```python
from build123d import *

# Parameters (mm, degrees)
SKETCH1_W                = 26.92
SKETCH1_H                = 12.7
BOSS_EXTRUDE1_DEPTH      = 4.95
BOSS_EXTRUDE1_DEPTH_BACK = 3.56
CUT_EXTRUDE1_DEPTH       = 9.51
SKETCH3_R                = 2.425
BOSS_EXTRUDE2_DEPTH      = 20.57
FILLET1_R                = 2.425
CHAMFER1_SIZE            = 0.5


with BuildPart() as part:
    # Sketch1 → Boss-Extrude1 (new body, two sides)
    with BuildSketch(Plane.XY) as boss_extrude1_sk:
        Rectangle(SKETCH1_W, SKETCH1_H)
    extrude(amount=BOSS_EXTRUDE1_DEPTH)
    extrude(boss_extrude1_sk.sketch, amount=-BOSS_EXTRUDE1_DEPTH_BACK)

    # Sketch2 → Cut-Extrude1 (cut, through all)
    with BuildSketch(Plane.XY.offset(4.95)):
        with BuildLine():
            Line((-12.065, 1.825), (-13.46, 1.825))
            ThreePointArc((-13.46, 1.825), (-14.425, 2.79), (-13.46, 3.755))
            Line((-13.46, 3.755), (-12.065, 3.755))
            ThreePointArc((-12.065, 3.755), (-11.1, 2.79), (-12.065, 1.825))
        make_face()
        with BuildLine():
            Line((12.065, 1.825), (13.46, 1.825))
            ThreePointArc((13.46, 1.825), (14.425, 2.79), (13.46, 3.755))
            Line((13.46, 3.755), (12.065, 3.755))
            ThreePointArc((12.065, 3.755), (11.1, 2.79), (12.065, 1.825))
        make_face()
    extrude(amount=-CUT_EXTRUDE1_DEPTH, mode=Mode.SUBTRACT)

    # Sketch3 → Boss-Extrude2 (add)
    with BuildSketch(Plane(origin=(13.46, 0, 0), x_dir=(0, 0, -1), z_dir=(1, 0, 0))):
        with Locations((0, -2.79)):
            Circle(SKETCH3_R)
    extrude(amount=BOSS_EXTRUDE2_DEPTH)

    # Fillet1
    fillet1_edges = [part.edges().sort_by_distance(p)[0] for p in [
        (34.03, -2.79, 2.425),
    ]]
    fillet(fillet1_edges, radius=FILLET1_R)

    # Chamfer1
    chamfer1_edges = [part.edges().sort_by_distance(p)[0] for p in [
        (13.46, 6.35, 0.695),
        (13.46, 5.0525, -3.56),
        (0, 6.35, -3.56),
        (-13.46, 6.35, 0.695),
        (13.46, 5.0525, 4.95),
        (0, 6.35, 4.95),
        (-13.46, 5.0525, 4.95),
        (13.46, -6.35, 0.695),
        (-13.46, -2.2625, -3.56),
        (13.46, -2.2625, -3.56),
        (0, -6.35, -3.56),
        (-13.46, -6.35, 0.695),
        (13.46, -2.2625, 4.95),
        (0, -6.35, 4.95),
        (-13.46, -2.2625, 4.95),
    ]]
    chamfer(chamfer1_edges, length=CHAMFER1_SIZE)


solid = part.part
```
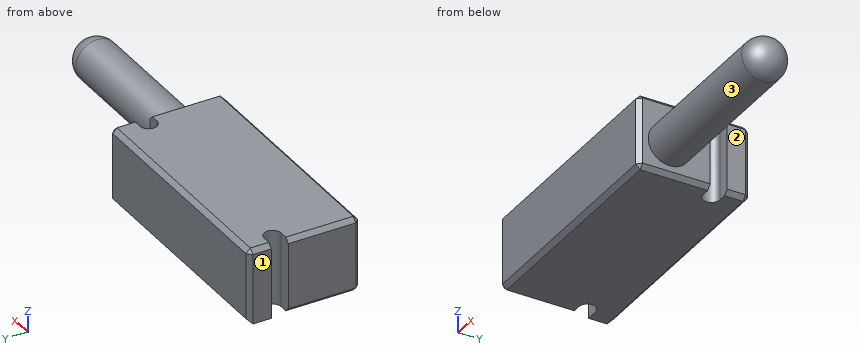
CAD build for the part. Positions are in the model's coordinates, mm. Face numbers are marked on the shaded views. A direction names the side the tool comes from. Round coordinates to 2 decimals unless told otherwise and drop trailing zeros. Order: outer loops, then holes, each group sorted by start corner. A loop starts at its lowest first (then second) coordinate and runs counter-clockwise, first axis right, second up. Notation, with made-up numbers: (19, 69.5) - (71, 69.5) arc R17 ccw to (71, 75.5) - close; hole circle Ø10 at (33.5, 40.25). An arc over 180 degrees is marked (long way). Answer in a Markdown table with one row per item. Add a question column.
(1) Probe L1, parallel to X at y = 4, z = 2; L2, parallel to Y at x = 25.5, z = 0 (3 decimals); L3, parallel to Z at x = 31.5, y = -3. List the from-to ranges inside material, lowest first. Write a range as [from, to].
(2) Band-saw the part on C-C on y = -2.79. List the corners of the cut face in (x, z) (3 decimals), and give its area (3 significant figures).
(3) Drop flat-ended pins along their axis: pin 1 Ø0.7 at (x, z) = (13, 1.5) entering from -Y; pin 2 Ø1.5 at (x, y) = (14, -1) entering from +Z; pin 3 Ø3 at (x, z) = (25, -1.5) entering from -Y (3 decimals); pin 4 Ø2.5 at (y, z) = (5, 0.5) entering from +X. Give the stop position or say it passes through.
(4) Band-saw the part on A-A on y = 0.5. List the corners of the cut face in (x, z), and give its area (3 significant figures).
(5) 3-axis set-ups, long thin cutter, end or side, ignore diameter. For the marked faces 1, 2 and 3: which of +Z, -Z, +X, -X, +Y, -Y reach the whole face in a straight line?
(6) Band-saw the part on D-D on z = 0. List the corners of the cut face in (x, y) (3 decimals), and give its area (3 significant figures).
(7) Band-saw the part on B-B on z = 3. List the corners of the cut face in (x, y) (3 decimals), and give its area (3 significant figures).
Data:
| question | item | result |
|---|---|---|
| 1 | L1 | x = [-13.46, 13.46] |
| 1 | L2 | y = [-5.215, -0.365] |
| 1 | L3 | z = [-2.42, 2.42] |
| 2 | outline | (-13.46, -3.06) - (-12.96, -3.56) - (12.96, -3.56) - (13.46, -3.06) - (13.46, -2.425) - (31.605, -2.425) arc R2.425 ccw to (31.605, 2.425) - (13.46, 2.425) - (13.46, 4.45) - (12.96, 4.95) - (-12.96, 4.95) - (-13.46, 4.45) - close |
| 2 | area | 326 mm^2 |
| 3 | pin 1 | stops at y = -6.35 |
| 3 | pin 2 | stops at z = 4.66 |
| 3 | pin 3 | stops at y = -5.215 |
| 3 | pin 4 | stops at x = 13.46 |
| 4 | outline | (-13.46, -3.06) - (-12.96, -3.56) - (12.96, -3.56) - (13.46, -3.06) - (13.46, 4.45) - (12.96, 4.95) - (-12.96, 4.95) - (-13.46, 4.45) - close |
| 4 | area | 229 mm^2 |
| 5 | face 1 | +Z, -Z, -X, +Y, -Y |
| 5 | face 2 | +Z, -Z, +X, +Y |
| 5 | face 3 | +X |
| 6 | outline | (-13.46, -5.85) - (-12.96, -6.35) - (12.96, -6.35) - (13.46, -5.85) - (13.46, -5.215) - (31.605, -5.215) arc R2.425 ccw to (31.605, -0.365) - (13.46, -0.365) - (13.46, 1.825) - (12.065, 1.825) arc R0.965 cw to (12.065, 3.755) - (13.46, 3.755) - (13.46, 5.85) - (12.96, 6.35) - (-12.96, 6.35) - (-13.46, 5.85) - (-13.46, 3.755) - (-12.065, 3.755) arc R0.965 cw to (-12.065, 1.825) - (-13.46, 1.825) - close |
| 6 | area | 430 mm^2 |
| 7 | outline | (-13.46, -5.85) - (-12.96, -6.35) - (12.96, -6.35) - (13.46, -5.85) - (13.46, 1.825) - (12.065, 1.825) arc R0.965 cw to (12.065, 3.755) - (13.46, 3.755) - (13.46, 5.85) - (12.96, 6.35) - (-12.96, 6.35) - (-13.46, 5.85) - (-13.46, 3.755) - (-12.065, 3.755) arc R0.965 cw to (-12.065, 1.825) - (-13.46, 1.825) - close |
| 7 | area | 333 mm^2 |
